from build123d import *

# Parameters (mm, degrees)
F0_W     = 9.525
F0_H     = 19.05
F0_R     = 1.190625
F1_DEPTH = 9.525
F2_W     = 6.35
F2_H     = 12.7
F3_DEPTH = 9.526


with BuildPart() as f1:
    # F0 (on Right) → F1 (new body)
    with BuildSketch(Plane.YZ):
        with Locations((-4.7625, 9.525)):
            Rectangle(F0_W, F0_H)
        with Locations((-4.7625, 6.35)):
            Circle(F0_R, mode=Mode.SUBTRACT)
        with Locations((-4.7625, 12.7)):
            Circle(F0_R, mode=Mode.SUBTRACT)
        with BuildLine():
            Line((-9.525, 19.05), (0, 19.05))
            Line((0, 19.05), (0, 25.4))
            ThreePointArc((0, 25.4), (-4.7625, 20.6375), (-9.525, 25.4))
            Line((-9.525, 25.4), (-9.525, 19.05))
        make_face()
        with BuildLine():
            ThreePointArc((-9.525, 25.4), (-4.7625, 20.6375), (0, 25.4))
            Line((0, 25.4), (-2.38125, 25.4))
            ThreePointArc((-2.38125, 25.4), (-4.7625, 23.01875), (-7.14375, 25.4))
            Line((-7.14375, 25.4), (-9.525, 25.4))
        make_face()
        with BuildLine():
            Line((-2.38125, 25.4), (0, 25.4))
            ThreePointArc((0, 25.4), (-4.7625, 30.1625), (-9.525, 25.4))
            Line((-9.525, 25.4), (-7.14375, 25.4))
            ThreePointArc((-7.14375, 25.4), (-4.7625, 27.78125), (-2.38125, 25.4))
        make_face()
    extrude(amount=F1_DEPTH)

    # F2 (on face) → F3 (cut, through all)
    with BuildSketch(Plane.XZ.offset(9.525)):
        with Locations((4.7625, 25.4)):
            Rectangle(F2_W, F2_H)
    extrude(amount=-F3_DEPTH, mode=Mode.SUBTRACT)


solid = f1.part
Input: part model. Units: mm. Frame: model coordinates. A direction names the side the tool comes from. Coordinates: 2 decimals unless noted, no trailing zeros. Order: outer loops, then holes, each group sorted by start corner. A loop starts at its lowest first (then second) coordinate and runs counter-clockwise, first axis right, second up. Notation, with made-up numbers: M 69,-8 L 125,-8 A15 cw 125,16 Z; hole C -29.75,47.5 d8. An arc over 180 degrees is marked long. One line per question, with ' | ' between items.
Item 1: Section B-B (x = 7). Give the number of separate pieces and of enclosed holes in the cut face, then the cut area to 3 significant figures.
Geometry results:
separate pieces: 1 | enclosed holes: 2 | area: 173 mm^2
Item 2: Draft query along X for faces 1 (the flat face through (5, -5, 19.05)), 2 (the cylindrical face through (4.696, -3.627, 13.058)), 3 (the flat face through (9.525, -5, 15)). Return one class per face: released by +X, released by -X, zero draft, split by the parting line, or undercut.
Geometry results:
face 1: undercut | face 2: zero draft | face 3: released by +X
Item 3: Section D-D (z = 25). Output: boundary loops of the cut face in (x, y) (1 decimal), then the cut area to 3 significant figures.
Geometry results:
outline: M 0,-9.5 L 1.6,-9.5 L 1.6,-7.1 L 0,-7.1 Z; M 0,-2.4 L 1.6,-2.4 L 1.6,0 L 0,0 Z; M 7.9,-9.5 L 9.5,-9.5 L 9.5,-7.1 L 7.9,-7.1 Z; M 7.9,-2.4 L 9.5,-2.4 L 9.5,0 L 7.9,0 Z | area: 15.3 mm^2
Item 4: Section A-A (z = 6.35). Output: boundary loops of the cut face in (x, y) (3 decimals).
Geometry results:
outline: M 0,-9.525 L 9.525,-9.525 L 9.525,-5.953 L 0,-5.953 Z; M 0,-3.572 L 9.525,-3.572 L 9.525,0 L 0,0 Z
Item 5: Ray query, line 1 along X through (y, z) = (-8.5, 20) (1 decimal); line 2 along Z through (x, y) = (4, -4); line 3 along Z through (x, y) = (8.75, -5.5). Return the intervals inside material, ascending.
Geometry results:
line 1: x = 0 to 1.6, 7.9 to 9.5 | line 2: z = 0 to 5.44, 7.26 to 11.79, 13.61 to 19.05 | line 3: z = 0 to 5.42, 7.28 to 11.77, 13.63 to 23.14, 27.66 to 30.11
Item 6: Reachability of faces 4 (the flat face through (7.938, -6, 23)), 5 (the flat face through (5, 0, 10)) from +Z, -Z, +X, -X, +Y, -Y: full face, straight path, thin tool, end or side. Return the list, or none.
Geometry results:
face 4: +Z, +Y, -Y | face 5: +Z, -Z, +X, -X, +Y
Item 7: Pin query (flat end, axial travel): pin 1 (1 mm diameter, centred on x = 8, y = -3, fed in from +Z); pin 2 (2 mm diameter, centred on x = 3, y = -3.5, fed in from +Z). Return the tip coordinate at first contact, or that it passes through.
Geometry results:
pin 1: stops at z = 29.99 | pin 2: stops at z = 19.05
